```python
from build123d import *

# Parameters (mm, degrees)
SKETCH_1_R          = 250
EXTRUDE_1_DEPTH     = 100
SKETCH_2_W          = 400
SKETCH_2_H          = 300
EXTRUDE_2_DEPTH     = 500
FILLET_1_R          = 150
FILLET_2_R          = 150
CUT_EXTRUDE_1_DEPTH = 250
SKETCH_4_R          = 100
CUT_EXTRUDE_2_DEPTH = 250


with BuildPart() as part:
    # 草图1 → 凸台-拉伸1 (new body)
    with BuildSketch(Plane(origin=(0, 0, 0), x_dir=(1, 0, 0), z_dir=(0, 1, 0))):
        with Locations(Location((0, 0, 0), (0, 0, 270))):
            Circle(SKETCH_1_R)
    extrude(amount=EXTRUDE_1_DEPTH)

    # 草图2 → 凸台-拉伸2 (add)
    with BuildSketch(Plane(origin=(0, 100, 0), x_dir=(1, 0, 0), z_dir=(0, 1, 0))):
        Rectangle(SKETCH_2_W, SKETCH_2_H)
    extrude(amount=EXTRUDE_2_DEPTH)

    # 圆角1
    fillet_1_edges = [part.edges().sort_by_distance(p)[0] for p in [
        (0, 600, 150),
    ]]
    fillet(fillet_1_edges, radius=FILLET_1_R)

    # 圆角2
    fillet_2_edges = [part.edges().sort_by_distance(p)[0] for p in [
        (0, 600, -150),
    ]]
    fillet(fillet_2_edges, radius=FILLET_2_R - 0.0001)  # a hair under: the kernel refuses the full size

    # 草图3 → 切除-拉伸1 (cut, symmetric)
    with BuildSketch(Plane.XY):
        Polygon((0, 600), (100, 600), (100, 270), (0, 270), (-100, 270), (-100, 600), align=None)
    extrude(amount=CUT_EXTRUDE_1_DEPTH, both=True, mode=Mode.SUBTRACT)

    # 草图4 → 切除-拉伸2 (cut, symmetric)
    with BuildSketch(Plane.XY):
        with Locations((0, 270)):
            Circle(SKETCH_4_R)
    extrude(amount=CUT_EXTRUDE_2_DEPTH, both=True, mode=Mode.SUBTRACT)


solid = part.part
```
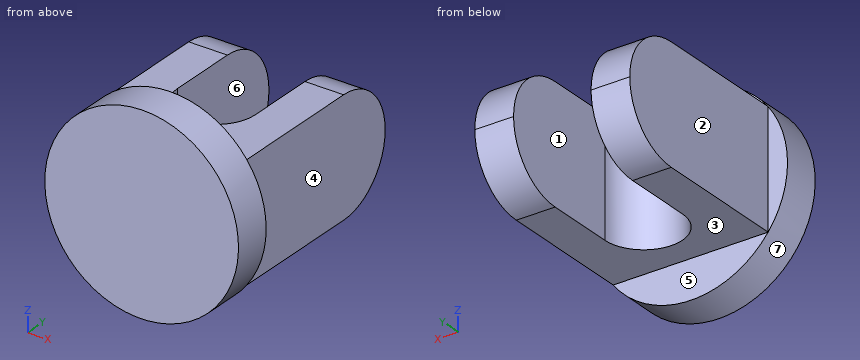
Can you work these out from the model? Positions are in its coordinate system, mm. Face numbers are marked on the shaded views. A direction names the side the tool comes from. Coordinates: 2 decimals unless noted, no trailing zeros. Loops run counter-clockwise (first coordinate to the right, second up) from the corner with the lowest first, then second, coordinate; pieces in that order, holes last.
1) Thinking about a two-plate mould opening in X: for the marked faces 5, 6 and 7, which applies, pulls with the +X half, pulls with the -X half, needs draft (parallel to the pull), parting line crosses it, or undercut?
2) I need wall thicknesses on probe 1 along X at (y, z) = (439, -118.5); probe 2 along Z at (x, y) = (-130.5, 267); probe 3 along Y at (x, z) = (-183.5, 2). Which ranges of each line are inside material? Lowest first, please.
3) For pin 1 (2 mm diameter, centred on y = 160.5, z = -92, fed in from +X); pin 2 (25 mm diameter, centred on x = 215.5, z = -25.5, fed in from +Y); pin 3 (12 mm diameter, centred on y = 177, z = 103, fed in from -X), each with a flat end and sliding along its axis, tell me the tip position at first contact or that it passes through.
4) Imagine slicing it at A-A on y = 344.5. List the corners of the cut face in (x, z) for me, plus the area to 3 significant figures.
5) Which directions (+Z, -Z, +X, -X, +Y, -Y) give clear straight access to the entire face, cutting with the end or side of a thin tool? Please do the marked faces 1, 2, 3 and 4.
6) Imagine slicing it at D-D on y = 87.5. List the corners of the cut face in (x, z) for me, plus the area to 3 significant figures.
7) Imagine slicing it at B-B on x = 0. List the corners of the cut face in (y, z) for me.
8) Imagine slicing it at C-C on z = -96. List the corners of the cut face in (x, y) for me, plus the area to 3 significant figures.
Completed:
1. face 5: needs draft
1. face 6: undercut
1. face 7: parting line crosses it
2. probe 1: x = -200 to -100, 100 to 200
2. probe 2: z = -150 to 150
2. probe 3: y = 0 to 599.99
3. pin 1: stops at x = 200
3. pin 2: stops at y = 100
3. pin 3: stops at x = -200
4. outline: (-200, -150) - (-100, -150) - (-100, 150) - (-200, 150) - close; (100, -150) - (200, -150) - (200, 150) - (100, 150) - close
4. area: 60,000 mm2
5. face 1: +Z, -Z, +Y
5. face 2: +Z, -Z, -X, +Y
5. face 3: -Z, +X, -X, +Y
5. face 4: +Z, -Z, +X, +Y
6. outline: circle Ø500 at (0, 0)
6. area: 196,000 mm2
7. outline: (0, -250) - (100, -250) - (100, -150) - (170, -150) - (170, 150) - (100, 150) - (100, 250) - (0, 250) - close
8. outline: (-230.83, 0) - (230.83, 0) - (230.83, 100) - (200, 100) - (200, 565.26) - (100, 565.26) - (100, 270) arc R100 cw to (-100, 270) - (-100, 565.26) - (-200, 565.26) - (-200, 100) - (-230.83, 100) - close
8. area: 158,000 mm2
